Build history of the part. All positions in model axes, mm. A direction names the side the tool comes from. Round coordinates to 2 decimals unless told otherwise and drop trailing zeros. Loops run counter-clockwise (first coordinate to the right, second up) from the corner with the lowest first, then second, coordinate; pieces in that order, holes last. Notation, with made-up numbers: (24.5, 36.5) -> (69.5, 36.5) arc R13 ccw to (69.5, 53.5) -> close; hole circle Ø11 at (-10, 72.25). An arc over 180 degrees is marked (long way). Put each result on its own line as item: value. Start each with the question number.
Item 1: Flat gauge pins, fed straight in: pin 1 Ø3 at (x, y) = (51, 14) entering from +Z; pin 2 Ø4 at (y, z) = (12.5, 20.5) entering from -X; pin 3 Ø23 at (y, z) = (-24, 0.5) entering from +X; pin 4 Ø10 at (x, z) = (41.5, 14) entering from +Y. Where does each tip first touch, or does it go through?
Item 2: Cut at A-A, the plane y = 0. List the corners of the cut face in (x, z).
Item 3: Tool access for faces 1 (the flat face through (25, 32, 0)), 2 (the flat face through (50, 0, -21)), 3 (the flat face through (19, 0, 11)), 4 (the flat face through (50, -21, 0)), 5 (the flat face through (81, 11, 0)): list every direction of +Z, -Z, +X, -X, +Y, -Y with a clear straight run to the whole face (end or side of a thin tool).
Item 4: Cut at C-C, the plane x = 115.5. List the corners of the cut face in (y, z).
Item 5: Cut at B-B, the plane z = 0. List the corners of the cut face in (x, y), plus the area to 3 significant figures.
Item 6: Cut at D-D, the plane z = -16.5. List the corners of the cut face in (x, y).
Item 7: Drill centre lines: probe 1 along X at (y, z) = (1.5, 0); probe 2 along X at (y, z) = (-4, 0); probe 3 along Y at (x, z) = (0, 5.5). Where is each one in solid material? Low to high. Write a range as [from, to].
Item 8: Pull direction Y, two halves, no side cores. Call faces 6 (the flat face through (19, 0, -11)), 7 (the cylindrical face through (-2.343, 17.847, -0.154)), 8 (the flat face through (25, -32, 0)), 9 (the cylindrical face through (-31.992, -0.704, 0.154)): +Y half, -Y half, draft (parallel to the pull), parting line (faces both ways), or undercut.
```python
from build123d import *

# Parameters (mm, degrees)
SKETCH1_R           = 18
BOSS_EXTRUDE1_DEPTH = 11
SKETCH2_R           = 18
BOSS_EXTRUDE2_DEPTH = 11


with BuildPart() as part:
    # Sketch1 → Boss-Extrude1 (new, symmetric)
    with BuildSketch(Plane.XY):
        with BuildLine():
            Line((0, 32), (50, 32))
            Line((50, 32), (50, -32))
            Line((50, -32), (0, -32))
            ThreePointArc((0, -32), (-32, 0), (0, 32))
        make_face()
        Circle(SKETCH1_R, mode=Mode.SUBTRACT)
    extrude(amount=BOSS_EXTRUDE1_DEPTH, both=True)

    # Sketch2 → Boss-Extrude2 (add, symmetric)
    with BuildSketch(Plane(origin=(100, 0, 0), x_dir=(-1, 0, 0), z_dir=(0, 1, 0))):
        with BuildLine():
            Line((0, 32), (50, 32))
            Line((50, 32), (50, -32))
            Line((50, -32), (0, -32))
            ThreePointArc((0, -32), (-32, 0), (0, 32))
        make_face()
        with Locations(Location((0, 0, 0), (0, 0, 90))):
            Circle(SKETCH2_R, mode=Mode.SUBTRACT)
    extrude(amount=BOSS_EXTRUDE2_DEPTH, both=True)


solid = part.part
```
Reply:
1. pin 1: stops at z = 11
1. pin 2: stops at x = 50
1. pin 3: stops at x = 50
1. pin 4: stops at y = 32
2. outline: (-32, -11) -> (-18, -11) -> (-18, 11) -> (-32, 11) -> close; (18, -11) -> (50, -11) -> (50, -32) -> (100, -32) arc R32 ccw to (100, 32) -> (50, 32) -> (50, 11) -> (18, 11) -> close; hole circle Ø36 at (100, 0)
3. face 1: +Z, -Z, +X, -X, +Y
3. face 2: -Z, -X, +Y, -Y
3. face 3: +Z, -X, +Y, -Y
3. face 4: +Z, -Z, +X, -Y
3. face 5: +Z, -Z, +X, +Y
4. outline: (-11, -28) -> (11, -28) -> (11, -9.15) -> (-11, -9.15) -> close; (-11, 9.15) -> (11, 9.15) -> (11, 28) -> (-11, 28) -> close
5. outline: (0, -32) -> (50, -32) -> (50, -11) -> (82, -11) -> (82, 11) -> (50, 11) -> (50, 32) -> (0, 32) arc R32 ccw to start; (118, -11) -> (132, -11) -> (132, 11) -> (118, 11) -> close; hole circle Ø36 at (0, 0)
5. area: 4,800 mm^2
6. outline: (50, -11) -> (92.81, -11) -> (92.81, 11) -> (50, 11) -> close; (107.19, -11) -> (127.42, -11) -> (127.42, 11) -> (107.19, 11) -> close
7. probe 1: x = [-31.96, -17.94], [17.94, 82], [118, 132]
7. probe 2: x = [-31.75, -17.55], [17.55, 82], [118, 132]
7. probe 3: y = [-32, -18], [18, 32]
8. face 6: draft
8. face 7: undercut
8. face 8: -Y half
8. face 9: parting line
